from build123d import *

# Parameters (mm, degrees)
BOSS_EXTRUDE1_DEPTH = 18.36
BOSS_EXTRUDE2_START = 16.01
SKETCH2_R           = 7.655
BOSS_EXTRUDE2_DEPTH = 16.01
SKETCH3_R           = 3.005
BOSS_EXTRUDE3_DEPTH = 3.56
SKETCH4_R           = 2
BOSS_EXTRUDE4_DEPTH = 21.2
CUT_EXTRUDE1_START  = -21.2
CUT_EXTRUDE1_DEPTH  = 21.2


with BuildPart() as part:
    # Sketch1 → Boss-Extrude1 (new body)
    with BuildSketch(Plane(origin=(0, 0, 0), x_dir=(0, 0, -1), z_dir=(1, 0, 0))):
        with BuildLine():
            Line((-5.9, 0), (-5.9, 4.87739941))
            ThreePointArc((-5.9, 4.87739941), (0, 7.655), (5.9, 4.87739941))
            Line((5.9, 4.87739941), (5.9, 0))
            Line((5.9, 0), (5.9, -4.87739941))
            ThreePointArc((5.9, -4.87739941), (0, -7.655), (-5.9, -4.87739941))
            Line((-5.9, -4.87739941), (-5.9, 0))
        make_face()
    extrude(amount=BOSS_EXTRUDE1_DEPTH)

    # Sketch2 → Boss-Extrude2 (add)
    with BuildSketch(Plane.ZY.offset(BOSS_EXTRUDE2_START)):
        Circle(SKETCH2_R)
    extrude(amount=-BOSS_EXTRUDE2_DEPTH)

    # Sketch3 → Boss-Extrude3 (add)
    with BuildSketch(Plane.ZY.offset(16.01)):
        Circle(SKETCH3_R)
    extrude(amount=BOSS_EXTRUDE3_DEPTH)

    # Sketch4 → Boss-Extrude4 (add)
    with BuildSketch(Plane.ZY.offset(19.57)):
        Circle(SKETCH4_R)
    extrude(amount=BOSS_EXTRUDE4_DEPTH)

    # Sketch5 → Cut-Extrude1 (cut)
    with BuildSketch(Plane.ZY.offset(40.77).offset(CUT_EXTRUDE1_START)):
        with BuildLine():
            Line((-1.5, -1.322875656), (-1.5, 0))
            Line((-1.5, 0), (-1.5, 1.322875656))
            ThreePointArc((-1.5, 1.322875656), (-2, 0), (-1.5, -1.322875656))
        make_face()
    extrude(amount=CUT_EXTRUDE1_DEPTH, mode=Mode.SUBTRACT)


solid = part.part
Source: CAD feature listing. Evaluate the final solid. Frame: model axes, mm. A direction names the side the tool comes from. Round coordinates to 2 decimals unless told otherwise and drop trailing zeros. Order: outer loops, then holes, each group sorted by start corner. A loop starts at its lowest first (then second) coordinate and runs counter-clockwise, first axis right, second up. Notation, with made-up numbers: (-23, -29.75) -> (6, -29.75) arc R20 ccw to (6, -19.75) -> close; hole circle Ø8 at (44.25, -28.5). An arc over 180 degrees is marked (long way). Answer as CSV lines item,"result".
Item 1: Line query: L1, parallel to Z at x = 9, y = 2.5; L2, parallel to X at y = 5, z = 2.75; L3, parallel to X at y = 1, z = -6.25. Output: solid intervals per line, ascending.
A:
L1,"-5.9 to 5.9"
L2,"-16.01 to 18.36"
L3,"-16.01 to 0"
Item 2: Section C-C, the plane x = -31. Return loops of the section in (y, z), plus the area to 3 significant figures.
A:
outline,"(-1.32, -1.5) -> (1.32, -1.5) arc R2 ccw (long way) to start"
area,"11.7 mm²"
Item 3: Section A-A, the plane z = 0. Return loops of the section in (x, y) (3 decimals), plus the area to 3 significant figures.
A:
outline,"(-40.77, -2) -> (-19.57, -2) -> (-19.57, -3.005) -> (-16.01, -3.005) -> (-16.01, -7.655) -> (18.36, -7.655) -> (18.36, 7.655) -> (-16.01, 7.655) -> (-16.01, 3.005) -> (-19.57, 3.005) -> (-19.57, 2) -> (-40.77, 2) -> close"
area,"632 mm²"
Item 4: Section D-D, the plane y = -5.5. Return loops of the section in (x, z), plus the area to 3 significant figures.
A:
outline,"(-16.01, -5.32) -> (18.36, -5.32) -> (18.36, 5.32) -> (-16.01, 5.32) -> close"
area,"366 mm²"
Item 5: Pin query (flat end, axial travel): pin 1 Ø0.5 at (y, z) = (2.5, -7) entering from +X; pin 2 Ø5 at (x, z) = (-12.5, -3.5) entering from -Y; pin 3 Ø5 at (x, y) = (10, 0.5) entering from +Z. Return the tip coordinate at first contact, or that it passes through.
A:
pin 1,"x = 0"
pin 2,"y = -7.59"
pin 3,"z = 5.9"
Item 6: Section B-B, the plane y = 0. Return loops of the section in (x, z) (3 decimals).
A:
outline,"(-40.77, -1.5) -> (-19.57, -1.5) -> (-19.57, -3.005) -> (-16.01, -3.005) -> (-16.01, -7.655) -> (0, -7.655) -> (0, -5.9) -> (18.36, -5.9) -> (18.36, 5.9) -> (0, 5.9) -> (0, 7.655) -> (-16.01, 7.655) -> (-16.01, 3.005) -> (-19.57, 3.005) -> (-19.57, 2) -> (-40.77, 2) -> close"
Item 7: Reachability of faces 1 (the face through (0, 0, -7)), 2 (the face through (-30, 0, -1.5)), 3 (the face through (-30, 0, 2)) from +Z, -Z, +X, -X, +Y, -Y: full face, straight path, thin tool, end or side. Return the list, or none.
A:
face 1,"-Z, +X, +Y, -Y"
face 2,"-Z, -X, +Y, -Y"
face 3,"-X"
